from build123d import *

# Parameters (mm, degrees)
EXTRUDE_THIN1_DEPTH = 436.5625
FILLET1_R           = 1.016


with BuildPart() as part:
    # Sketch1 → Extrude-Thin1 (new body)
    with BuildSketch(Plane.XY):
        with BuildLine():
            Line((9.781263434, 50.00625), (1.15875723, 47.010410758))
            ThreePointArc((1.15875723, 47.010410758), (0.024053154, 45.094051318), (1.724851264, 43.65625))
            Line((1.724851264, 43.65625), (10.31875, 43.65625))
            Line((10.31875, 43.65625), (14.273529908, 42.8625))
            Line((14.273529908, 42.8625), (17.712331019, 32.965078439))
            ThreePointArc((17.712331019, 32.965078439), (19.450830911, 30.647054561), (22.211029908, 29.765625))
            Line((22.211029908, 29.765625), (23.798529908, 29.765625))
            Line((23.798529908, 29.765625), (23.798529908, 20.240625))
            Line((23.798529908, 20.240625), (43.65625, 20.240625))
            Line((43.65625, 20.240625), (43.65625, 17.065625))
            Line((43.65625, 17.065625), (37.30625, 16.271875))
            Line((37.30625, 16.271875), (37.30625, 13.890625))
            Line((37.30625, 13.890625), (34.13125, 13.890625))
            ThreePointArc((34.13125, 13.890625), (28.010554633, 12.880569241), (22.538913712, 9.957510902))
            ThreePointArc((22.538913712, 9.957510902), (17.520243065, 7.276438204), (11.90625, 6.35))
            Line((11.90625, 6.35), (10.31875, 6.35))
            Line((10.31875, 6.35), (1.724851264, 6.35))
            ThreePointArc((1.724851264, 6.35), (0.024053154, 4.912198682), (1.15875723, 2.995839242))
            Line((1.15875723, 2.995839242), (9.781263434, 0))
            Line((9.781263434, 0), (9.447813501, -0.95972243))
            Line((9.447813501, -0.95972243), (0.825307297, 2.036116813))
            ThreePointArc((0.825307297, 2.036116813), (-0.977778666, 5.081281519), (1.724851264, 7.366))
            Line((1.724851264, 7.366), (10.31875, 7.366))
            Line((10.31875, 7.366), (11.90625, 7.366))
            ThreePointArc((11.90625, 7.366), (17.193805978, 8.238568564), (21.920655776, 10.763744817))
            ThreePointArc((21.920655776, 10.763744817), (27.684117546, 13.842699601), (34.13125, 14.906625))
            Line((34.13125, 14.906625), (36.29025, 14.906625))
            Line((36.29025, 14.906625), (36.29025, 17.168781734))
            Line((36.29025, 17.168781734), (42.64025, 17.962531734))
            Line((42.64025, 17.962531734), (42.64025, 19.224625))
            Line((42.64025, 19.224625), (22.782529908, 19.224625))
            Line((22.782529908, 19.224625), (22.782529908, 28.749625))
            Line((22.782529908, 28.749625), (22.211029908, 28.749625))
            ThreePointArc((22.211029908, 28.749625), (18.861988459, 29.819092868), (16.752608589, 32.631628506))
            Line((16.752608589, 32.631628506), (13.504357649, 41.98061609))
            Line((13.504357649, 41.98061609), (10.217797732, 42.64025))
            Line((10.217797732, 42.64025), (1.724851264, 42.64025))
            ThreePointArc((1.724851264, 42.64025), (-0.977778666, 44.924968481), (0.825307297, 47.970133187))
            Line((0.825307297, 47.970133187), (9.447813501, 50.96597243))
            Line((9.447813501, 50.96597243), (9.781263434, 50.00625))
        make_face()
    extrude(amount=-EXTRUDE_THIN1_DEPTH)

    # Fillet1
    fillet1_edges = [part.edges().sort_by_distance(p)[0] for p in [
        (36.29025, 17.168781734, -218.28125),
        (22.782529908, 19.224625, -218.28125),
        (10.31875, 43.65625, -218.28125),
        (14.273529908, 42.8625, -218.28125),
        (23.798529908, 29.765625, -218.28125),
        (43.65625, 20.240625, -218.28125),
        (43.65625, 17.065625, -218.28125),
        (37.30625, 13.890625, -218.28125),
    ]]
    fillet(fillet1_edges, radius=FILLET1_R)


with BuildPart() as body_2:
    # Mirror1: mirrored copy
    add(part.part.mirror(Plane(origin=(0, 0, 0), x_dir=(0, 0, 1), z_dir=(1, 0, 0))))


solid = body_2.part
The model under review builds one solid part; all positions refer to its coordinate system, in mm. A direction names the side the tool comes from. Round coordinates to 2 decimals unless told otherwise and drop trailing zeros. Loops run counter-clockwise (first coordinate to the right, second up) from the corner with the lowest first, then second, coordinate; pieces in that order, holes last. Notation, with made-up numbers: (5, 0.5) -> (46, 0.5) arc R22 cw to (46, 29.5) -> close; hole circle Ø3 at (-17, -14). An arc over 180 degrees is marked (long way). One line per question, with ' | ' between items. Start each with the question number.
Item 1: Machinability: for faces 1 (the face through (-33, 20.241, -215)), 2 (the face through (-5.41, 1.52, -215.23)), 3 (the face through (-22.783, 24, -215)), 4 (the face through (-23, 21, 0)), 5 (the face through (-23, 21, -436.562)), which of the approach directions +Z, -Z, +X, -X, +Y, -Y give a long, thin tool a straight path to every point of the face, cutting with its end or side? Answer none if there is none.
Item 2: Add section A-A, the plane x = -5.5. Write out the cut boundary in (y, z), then the cut area to 3 significant figures.
Item 3: Add section B-B, the plane x = -29. Write out the cut boundary in (y, z), then the cut area to 3 significant figures.
Item 4: Wall thickness on line 1 along Y through (x, z) = (-35, -147.5); line 2 along Y through (x, z) = (-5, -247); line 3 along X through (y, z) = (26, -176): over which ranges is each line inside the solid? List them lowest first. Write a range as [from, to].
Item 5: For pin 1 (11 mm diameter, centred on x = -6.5, z = -272, fed in from -Y); pin 2 (4.5 mm diameter, centred on y = 26, z = -145, fed in from +X); pin 3 (9.5 mm diameter, centred on x = -32.5, z = -307, fed in from +Y), all flat-tipped, find the tip position at first contact; note any pin that passes through.
Item 6: Add section C-C, the plane y = 25. Write out the cut boundary in (x, z), then the cut area to 3 significant figures.
Return value:
1) face 1: +Z, -Z, -X, +Y | face 2: +Z, -Z, -X | face 3: +Z, -Z, +X | face 4: +Z, +X, -X, +Y, -Y | face 5: -Z, +X, -X, +Y, -Y
2) outline: (0.41, -436.56) -> (1.49, -436.56) -> (1.49, 0) -> (0.41, 0) -> close; (6.35, -436.56) -> (7.37, -436.56) -> (7.37, 0) -> (6.35, 0) -> close; (42.64, -436.56) -> (43.66, -436.56) -> (43.66, 0) -> (42.64, 0) -> close; (48.52, -436.56) -> (49.59, -436.56) -> (49.59, 0) -> (48.52, 0) -> close | area: 1,830 mm2
3) outline: (13.19, -436.56) -> (14.24, -436.56) -> (14.24, 0) -> (13.19, 0) -> close; (19.22, -436.56) -> (20.24, -436.56) -> (20.24, 0) -> (19.22, 0) -> close | area: 903 mm2
4) line 1: y = [13.89, 14.91], [19.22, 20.24] | line 2: y = [0.59, 1.66], [6.35, 7.37], [42.64, 43.66], [48.35, 49.42] | line 3: x = [-23.8, -22.78]
5) pin 1: stops at y = -0.96 | pin 2: stops at x = -22.78 | pin 3: stops at y = 20.24
6) outline: (-23.8, -436.56) -> (-22.78, -436.56) -> (-22.78, 0) -> (-23.8, 0) -> close | area: 444 mm2
